Could you check a few things on this model? Use its own coordinates, in mm. Face numbers are marked on the shaded views. A direction names the side the tool comes from. Give positions to 0.01 mm unless a question says otherwise; leave off trailing zeros. Loops run counter-clockwise (first coordinate to the right, second up) from the corner with the lowest first, then second, coordinate; pieces in that order, holes last. Notation, with made-up numbers: (19.25, -3) -> (60.25, -3) arc R23 ccw to (60.25, 11) -> close; hole circle Ø7 at (80, 36.5). An arc over 180 degrees is marked (long way). Put each result on its own line as item: value.
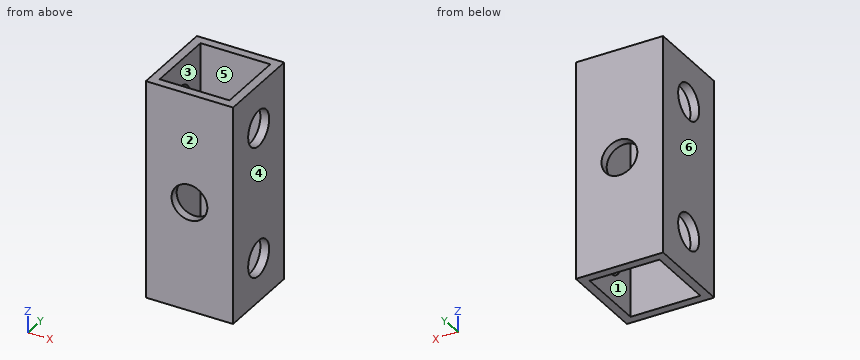
```python
from build123d import *

# Parameters (mm, degrees)
SKETCH_1_W          = 10
SKETCH_1_H          = 10
SKETCH_1_W_2        = 8
SKETCH_1_H_2        = 8
EXTRUDE_1_DEPTH     = 12.5
SKETCH_2_R          = 2.05
CUT_EXTRUDE_1_DEPTH = 11
SKETCH_3_R          = 2.05
CUT_EXTRUDE_2_DEPTH = 11


with BuildPart() as part:
    # 草图1 → 凸台-拉伸1 (new body, symmetric)
    with BuildSketch(Plane.XY):
        Rectangle(SKETCH_1_W, SKETCH_1_H)
        Rectangle(SKETCH_1_W_2, SKETCH_1_H_2, mode=Mode.SUBTRACT)
    extrude(amount=EXTRUDE_1_DEPTH, both=True)

    # 草图2 → 切除-拉伸1 (cut, through all)
    with BuildSketch(Plane(origin=(0, 5, 0), x_dir=(1, 0, 0), z_dir=(0, 1, 0))):
        Circle(SKETCH_2_R)
    extrude(amount=-CUT_EXTRUDE_1_DEPTH, mode=Mode.SUBTRACT)

    # 草图3 → 切除-拉伸2 (cut, through all)
    with BuildSketch(Plane(origin=(5, 0, 0), x_dir=(0, 0, -1), z_dir=(1, 0, 0))):
        with Locations((-7.5, 0)):
            Circle(SKETCH_3_R)
        with Locations((7.5, 0)):
            Circle(SKETCH_3_R)
    extrude(amount=-CUT_EXTRUDE_2_DEPTH, mode=Mode.SUBTRACT)


solid = part.part
```
1. If we section it at A-A (x = 0): List the corners of the cut face in (y, z) for me, then the cut area to 3 significant figures.
Recorded:
outline: (-5, -12.5) -> (-4, -12.5) -> (-4, -2.05) -> (-5, -2.05) -> close; (-5, 2.05) -> (-4, 2.05) -> (-4, 12.5) -> (-5, 12.5) -> close; (4, -12.5) -> (5, -12.5) -> (5, -2.05) -> (4, -2.05) -> close; (4, 2.05) -> (5, 2.05) -> (5, 12.5) -> (4, 12.5) -> close
area: 41.8 mm^2
2. Thinking about a two-plate mould opening in X: for the marked faces 1, 2, 3 and 4, which applies, pulls with the +X half, pulls with the -X half, needs draft (parallel to the pull), parting line crosses it, or undercut?
Recorded:
face 1: undercut
face 2: needs draft
face 3: undercut
face 4: pulls with the +X half
3. If we section it at B-B (x = -3.75): List the corners of the cut face in (y, z) for me, then the cut area to 3 significant figures.
Recorded:
outline: (-5, -12.5) -> (-4, -12.5) -> (-4, 12.5) -> (-5, 12.5) -> close; (4, -12.5) -> (5, -12.5) -> (5, 12.5) -> (4, 12.5) -> close
area: 50.0 mm^2
4. For the marked faces 5 and 6, which set-ups out of +Z, -Z, +X, -X, +Y, -Y let a thin tool reach every point of the face, with its end or its side?
Recorded:
face 5: +Z, -Z
face 6: +Z, -Z, -X, +Y, -Y
5. If we section it at C-C (z = 7.5): List the corners of the cut face in (x, y) for me.
Recorded:
outline: (-5, -5) -> (5, -5) -> (5, -2.05) -> (4, -2.05) -> (4, -4) -> (-4, -4) -> (-4, -2.05) -> (-5, -2.05) -> close; (-5, 2.05) -> (-4, 2.05) -> (-4, 4) -> (4, 4) -> (4, 2.05) -> (5, 2.05) -> (5, 5) -> (-5, 5) -> close
6. I need wall thicknesses on line 1 (X direction, y = 3.5, z = 11); line 2 (Y direction, x = -4.8, z = -7.5). Which ranges of each line are inside material? Lowest first, please.
Recorded:
line 1: x = -5 to -4, 4 to 5
line 2: y = -5 to -2.05, 2.05 to 5
